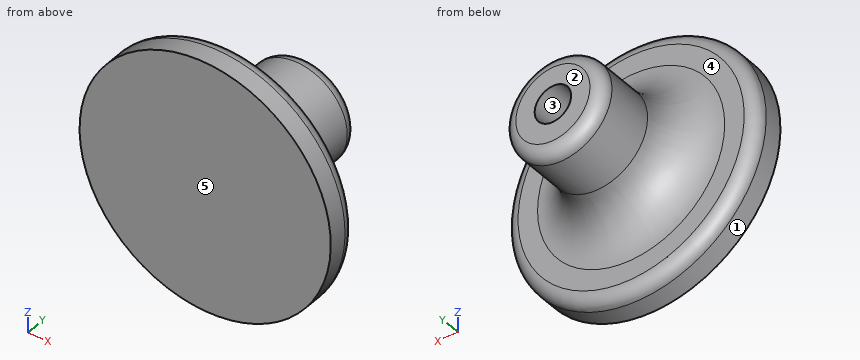
```python
from build123d import *


with BuildPart() as part:
    # Sketch2 → Revolve1 (revolve)
    with BuildSketch(Plane(origin=(0, 0, 0), x_dir=(0, 0, -1), z_dir=(1, 0, 0)), mode=Mode.PRIVATE) as revolve1_sk:
        with BuildLine():
            Line((0, 0), (-20, 0))
            Line((-20, 0), (-20, 3))
            ThreePointArc((-20, 3), (-19.414213562, 4.414213562), (-18, 5))
            Line((-18, 5), (-14.9, 5))
            ThreePointArc((-14.9, 5), (-9.950252532, 7.050252532), (-7.9, 12))
            Line((-7.9, 12), (-7.9, 19.5))
            ThreePointArc((-7.9, 19.5), (-7.314213562, 20.914213562), (-5.9, 21.5))
            Line((-5.9, 21.5), (-2.9, 21.5))
            Line((-2.9, 21.5), (-2.9, 1.5))
            Line((-2.9, 1.5), (0, 1.5))
            Line((0, 1.5), (0, 0))
        make_face()
    revolve(revolve1_sk.sketch.rotate(Axis((0, 0, 0), (0, 1, 0)), 180), axis=Axis((0, 0, 0), (0, 1, 0)))


solid = part.part
```
CAD build for the part. Positions are in the model's coordinates, mm. Face numbers are marked on the shaded views. A direction names the side the tool comes from. Give positions to 0.01 mm unless a question says otherwise; leave off trailing zeros. Order: outer loops, then holes, each group sorted by start corner. A loop starts at its lowest first (then second) coordinate and runs counter-clockwise, first axis right, second up.
(1) Saw through at A-A, the plane x = 0. Give the cut face in (y, z).
(2) Saw through at D-D, the plane y = 7. Give the cut face in (x, z), then the cut area to 3 significant figures.
(3) Tool access for the marked faces 4 and 5: list every direction of +Z, -Z, +X, -X, +Y, -Y with a clear straight run to the whole face (end or side of a thin tool).
(4) Saw through at C-C, the plane y = 10.75. Give the cut face in (x, z).
(5) Drill centre lines: L1, parallel to X at y = 13.5, z = 0; L2, parallel to Y at x = -14, z = 5; L3, parallel to Z at x = 2.5, y = 10. Where is each one in solid material? Low to high.
(6) Flat gauge pins, fed straight in: pin 1 (4 mm diameter, centred on y = 13, z = -2, fed in from +X); pin 2 (3 mm diameter, centred on x = -8.5, y = 12, fed in from +Z); pin 3 (2 mm diameter, centred on x = -5, y = 17, fed in from +Z). Where does each tip first touch, or does it go through?
(7) Saw through at B-B, the plane z = 0. Give the cut face in (x, y).
(8) Mould opens along X. For the marked faces 1, 2 and 3 say: released by +X, released by -X, zero draft, split by the parting line, or undercut.
Results found:
1. outline: (0, -20) - (3, -20) arc R2 ccw to (5, -18) - (5, -14.9) arc R7 cw to (12, -7.9) - (19.5, -7.9) arc R2 ccw to (21.5, -5.9) - (21.5, -2.9) - (1.5, -2.9) - (1.5, 2.9) - (21.5, 2.9) - (21.5, 5.9) arc R2 ccw to (19.5, 7.9) - (12, 7.9) arc R7 cw to (5, 14.9) - (5, 18) arc R2 ccw to (3, 20) - (0, 20) - close
2. outline: circle Ø20 at (0, 0); hole circle Ø5.8 at (0, 0)
2. area: 288 mm2
3. face 4: +Y
3. face 5: +Z, -Z, +X, -X, -Y
4. outline: circle Ø16.03 at (0, 0); hole circle Ø5.8 at (0, 0)
5. L1: x = -7.9 to -2.9, 2.9 to 7.9
5. L2: y = 0 to 5
5. L3: z = -7.8 to -1.47, 1.47 to 7.8
6. pin 1: stops at x = 7.9
6. pin 2: stops at z = 3.66
6. pin 3: stops at z = 6.81
7. outline: (-20, 0) - (20, 0) - (20, 3) arc R2 ccw to (18, 5) - (14.9, 5) arc R7 cw to (7.9, 12) - (7.9, 19.5) arc R2 ccw to (5.9, 21.5) - (2.9, 21.5) - (2.9, 1.5) - (-2.9, 1.5) - (-2.9, 21.5) - (-5.9, 21.5) arc R2 ccw to (-7.9, 19.5) - (-7.9, 12) arc R7 cw to (-14.9, 5) - (-18, 5) arc R2 ccw to (-20, 3) - close
8. face 1: split by the parting line
8. face 2: zero draft
8. face 3: undercut
